Design review of the part built by this model. Coordinates are the model's own, in mm. A direction names the side the tool comes from. Coordinates: 2 decimals unless noted, no trailing zeros. Write each loop counter-clockwise with the first axis right and the second up, starting at its lowest first coordinate (ties: lowest second). Pieces come first, ordered by that corner, then holes. Notation, with made-up numbers: (-31.75, 49.25) -> (-16.75, 49.25) arc R9 ccw to (-16.75, 65.25) -> close; hole circle Ø8 at (-9.75, -39). An arc over 180 degrees is marked (long way). Return JSON: item names as keys, results as strings. Group by question number.
from build123d import *

# Parameters (mm, degrees)
F0_W     = 25
F0_H     = 25
F1_DEPTH = 190
F2_T     = -2.5
F4_D     = 10
F5_D     = 5


with BuildPart() as f1:
    # F0 (on Front) → F1 (new body)
    with BuildSketch(Plane.XZ):
        with Locations((12.5, 12.5)):
            Rectangle(F0_W, F0_H)
    extrude(amount=-F1_DEPTH)

    # F2
    f2_openings = [f1.faces().sort_by_distance(p)[0] for p in [
        (12.5, 0, 12.5),
        (12.5, 190, 12.5),
    ]]
    offset(amount=F2_T, openings=f2_openings)

    # F4 (through all)
    with Locations(Plane.XY.offset(25)):
        with Locations((13.7, 156)):
            Hole(F4_D / 2)

    # F5 (through all)
    with Locations(Plane.XY.offset(25)):
        with Locations((13.7, 138), (13.7, 174)):
            Hole(F5_D / 2)


solid = f1.part
Q1. Wall thickness on L1, parallel to Y at x = 13.7, z = 23.85; L2, parallel to Z at x = 5.5, y = 33.5: over which ranges is each line inside the solid? List them lowest first.
Q2. We need section C-C on x = 13.7. State how many separate pieces and enclosed holes the cut face has, plus the area to 3 significant figures.
Q3. For faces 1 (the flat face through (0, 94, 12)), 2 (the flat face through (22.5, 94, 12)), list the 3-axis set-ups (+Z, -Z, +X, -X, +Y, -Y) from which the entire face can be reached by the end or side of a thin tool; tool diameter is ignored.
Q4. We need section B-B on z = 8. Write out the cut boundary in (x, y).
Q5. We need section A-A on y = 174. Write out the cut boundary in (x, z).
Q6. The part is to be moulded in two halves that separate along Y. For faces 3 (the cylindrical face through (14.03, 176.48, 1.23)), 4 (the flat face through (23, 0, 13)), 5 (the flat face through (12, 94, 25)), say which applies: +Y half, -Y half, draft (parallel to the pull), parting line (faces both ways), or undercut.
Q7. We need section D-D on y = 97.5. Write out the cut boundary in (x, z), plus the area to 3 significant figures.
Findings below:
{
 "1": {"L1": "y = 0 to 135.5, 140.5 to 151, 161 to 171.5, 176.5 to 190", "L2": "z = 0 to 2.5, 22.5 to 25"},
 "2": {"separate pieces": "8", "enclosed holes": "0", "area": "850 mm^2"},
 "3": {"face 1": "+Z, -Z, -X, +Y, -Y", "face 2": "+Y, -Y"},
 "4": {"outline": "(0, 0) -> (2.5, 0) -> (2.5, 190) -> (0, 190) -> close; (22.5, 0) -> (25, 0) -> (25, 190) -> (22.5, 190) -> close"},
 "5": {"outline": "(0, 0) -> (11.2, 0) -> (11.2, 2.5) -> (2.5, 2.5) -> (2.5, 22.5) -> (11.2, 22.5) -> (11.2, 25) -> (0, 25) -> close; (16.2, 0) -> (25, 0) -> (25, 25) -> (16.2, 25) -> (16.2, 22.5) -> (22.5, 22.5) -> (22.5, 2.5) -> (16.2, 2.5) -> close"},
 "6": {"face 3": "undercut", "face 4": "-Y half", "face 5": "draft"},
 "7": {"outline": "(0, 0) -> (25, 0) -> (25, 25) -> (0, 25) -> close; hole (2.5, 2.5) -> (22.5, 2.5) -> (22.5, 22.5) -> (2.5, 22.5) -> close", "area": "225 mm^2"}
}
